```python
from build123d import *

# Parameters (mm, degrees)
F1_DEPTH      = 25.4
F2_W          = 15.24
F2_H          = 27.5789452819
F3_DEPTH      = 9.526
F3_DEPTH_BACK = 9.526


with BuildPart() as f1:
    # F0 (on Front) → F1 (new body)
    with BuildSketch(Plane.XZ):
        with BuildLine():
            Line((3.6874021567, 9.525), (9.525, 9.525))
            ThreePointArc((9.525, 9.525), (0, 19.05), (-9.525, 9.525))
            Line((-9.525, 9.525), (-3.6874021567, 9.525))
            ThreePointArc((-3.6874021567, 9.525), (0, 13.2124021567), (3.6874021567, 9.525))
        make_face()
        with BuildLine():
            Line((9.525, -9.525), (9.525, 9.525))
            ThreePointArc((9.525, 9.525), (0, 0), (-9.525, 9.525))
            Line((-9.525, 9.525), (-9.525, -9.525))
            Line((-9.525, -9.525), (9.525, -9.525))
        make_face()
        with BuildLine():
            ThreePointArc((-9.525, 9.525), (0, 0), (9.525, 9.525))
            Line((9.525, 9.525), (3.6874021567, 9.525))
            ThreePointArc((3.6874021567, 9.525), (0, 5.8375978433), (-3.6874021567, 9.525))
            Line((-3.6874021567, 9.525), (-9.525, 9.525))
        make_face()
    extrude(amount=F1_DEPTH)

    # F2 (on Right) → F3 (cut, two sides)
    with BuildSketch(Plane.YZ) as f3_sk:
        with Locations((-12.7, 9.344472641)):
            Rectangle(F2_W, F2_H)
    extrude(amount=F3_DEPTH, mode=Mode.SUBTRACT)
    extrude(f3_sk.sketch, amount=-F3_DEPTH_BACK, mode=Mode.SUBTRACT)


solid = f1.part
```
The listing builds one solid part. Answer for the finished solid, in the listing's coordinates (mm). A direction names the side the tool comes from. Round coordinates to 2 decimals unless told otherwise and drop trailing zeros. Order: outer loops, then holes, each group sorted by start corner. A loop starts at its lowest first (then second) coordinate and runs counter-clockwise, first axis right, second up. Notation, with made-up numbers: (11, -25) - (18, -25) arc R24 ccw to (18, -3) - close; hole circle Ø9 at (5.5, 25.5). An arc over 180 degrees is marked (long way). Put each result on its own line as item: value. Start each with the question number.
(1) Find section D-D (z = 11.5). Give the vertices of the cut face in (x, y).
(2) Find section A-A (z = 3). Give the vertices of the cut face in (x, y) (3 decimals), plus the area to 3 significant figures.
(3) Find section C-C (y = -21.25). Give the vertices of the cut face in (x, z) (3 decimals), plus the area to 3 significant figures.
(4) Straight lines are drawn through the part: probe 1 along Y at (x, z) = (8.25, 5); probe 2 along Z at (x, y) = (0, -22.4) (3 decimals); probe 3 along Z at (x, y) = (-6.75, -19) (3 decimals). For each, find the intervals that lie inside material, in ascending order. Write a range as from..to.
(5) Determine the mould class of faces 1 (the flat face through (-9.525, -13, -6)), 2 (the cylindrical face through (-0.48, -22.82, 5.87)), 3 (the flat face through (0, -13, -4.445)) for opening direction X: released by +X, released by -X, zero draft, split by the parting line, or undercut.
(6) Given P1, Ø9.5, axis at x = 2, z = 8, coming from the -Y side; P2, Ø4.5, axis at x = 4.5, y = -13, coming from the +Z side (3 decimals); P3, Ø5, axis at x = -7, y = -19.5, coming from the +Z side, each flat-ended and moving along its own axis, determine where each tip first touches the part or whether it passes through.
(7) Find section B-B (x = 0). Give the vertices of the cut face in (y, z) (3 decimals).
(8) For faces 4 (the flat face through (9.525, -13, -6)), 5 (the flat face through (0, -5.08, 5)), determine the directions among +Z, -Z, +X, -X, +Y, -Y from which every point of the face is accessible in a straight line to the end or side of a thin tool.
Reply:
1. outline: (-9.32, -25.4) - (-3.11, -25.4) - (-3.11, -20.32) - (-9.32, -20.32) - close; (-9.32, -5.08) - (-3.11, -5.08) - (-3.11, 0) - (-9.32, 0) - close; (3.11, -25.4) - (9.32, -25.4) - (9.32, -20.32) - (3.11, -20.32) - close; (3.11, -5.08) - (9.32, -5.08) - (9.32, 0) - (3.11, 0) - close
2. outline: (-9.525, -25.4) - (9.525, -25.4) - (9.525, -20.32) - (-9.525, -20.32) - close; (-9.525, -5.08) - (9.525, -5.08) - (9.525, 0) - (-9.525, 0) - close
2. area: 194 mm^2
3. outline: (-9.525, -9.525) - (9.525, -9.525) - (9.525, 9.525) arc R9.525 ccw to (-9.525, 9.525) - close; hole circle Ø7.375 at (0, 9.525)
3. area: 463 mm^2
4. probe 1: -25.4..-20.32, -5.08..0
4. probe 2: -9.525..5.838, 13.212..19.05
4. probe 3: -9.525..-4.445
5. face 1: released by -X
5. face 2: undercut
5. face 3: zero draft
6. P1: y = -25.4
6. P2: z = -4.445
6. P3: z = 17.84
7. outline: (-25.4, -9.525) - (0, -9.525) - (0, 5.838) - (-5.08, 5.838) - (-5.08, -4.445) - (-20.32, -4.445) - (-20.32, 5.838) - (-25.4, 5.838) - close; (-25.4, 13.212) - (-20.32, 13.212) - (-20.32, 19.05) - (-25.4, 19.05) - close; (-5.08, 13.212) - (0, 13.212) - (0, 19.05) - (-5.08, 19.05) - close
8. face 4: +Z, -Z, +X, +Y, -Y
8. face 5: +Z, +X, -X
